Can you work these out from the drawing? Everything is in mm from the part's minimum corner. A direction names the side the tool comes from. Give positions to 0.01 mm unless a question says otherwise; leave off trailing zeros. Loops run counter-clockwise (first coordinate to the right, second up) from the corner with the lowest first, then second, coordinate; pieces in that order, holes last. Notation, with made-up numbers: (48, 48) -> (82, 48) arc R6 cw to (82, 52) -> close; hole circle Ø10 at (33.5, 2.5). An arc over 180 degrees is marked (long way). Write item = value, one per line. Start each with the question number.
1) I want a section at A-A (y = 2). List the corners of the cut face in (x, z) for me.
2) I want a section at B-B (x = 10). List the corners of the cut face in (y, z) for me, and give its area (3 significant figures).
3) I'm going to push flat-ended pins straight in: pin 1 Ø12 at (x, z) = (41.5, 8) entering from -Y; pin 2 Ø0.9 at (y, z) = (1.5, 19) entering from +X. Where does each tip first touch, or does it pass through?
4) On a 3-axis mill with a long thin cutter (end or side, diameter ignored), from which of +Z, -Z, +X, -X, +Y, -Y can I reach the whole of each face in a straight line? I mean the marked faces 1, 2 and 3. Say none if no direction works.
5) If we mould it in two halves opening along X, with no side actions, what happens to the marked faces 4, 5, 6 and 7? For each: +X half, -X half, draft (parallel to the pull), parting line (faces both ways), or undercut.
6) I need wall thicknesses on probe 1 along X at (y, z) = (0.35, 6); probe 2 along Z at (x, y) = (8, 0.9); probe 3 along Z at (x, y) = (39.5, 2.25). Which ranges of each line are inside material? Lowest first, please. Write a range as from..to.
7) I want a section at C-C (z = 22). List the corners of the cut face in (x, y) for me, and give its area (3 significant figures).
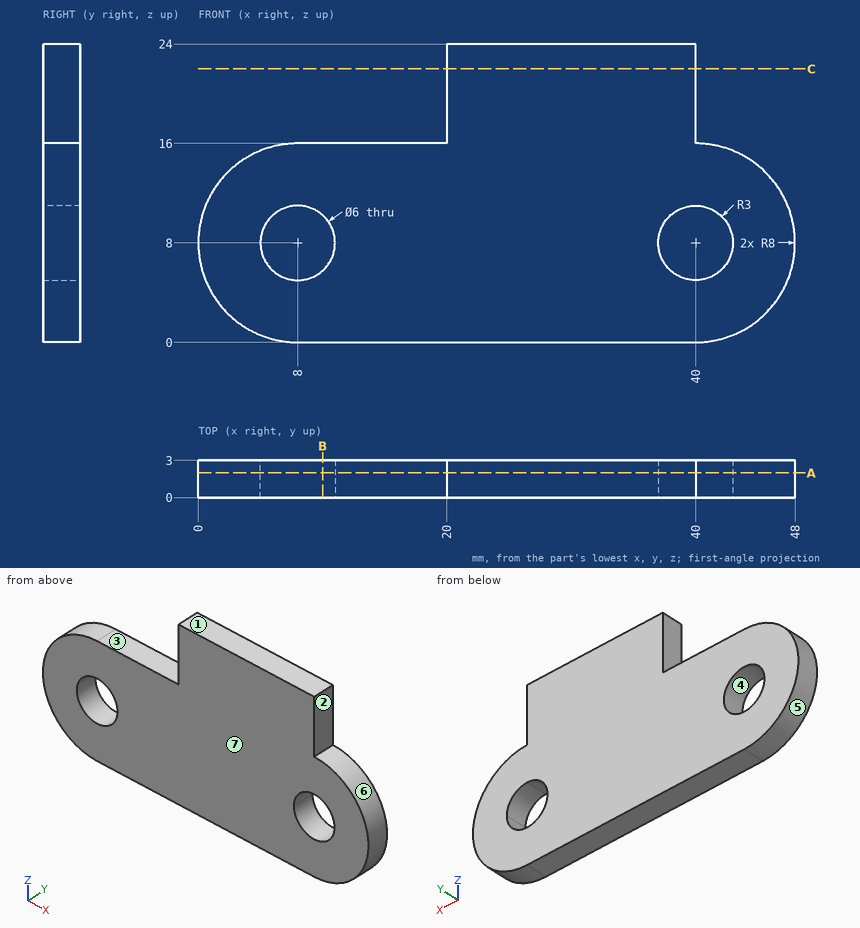
Answer list:
q1.outline = (8, 0) -> (40, 0) arc R8 ccw to (40, 16) -> (40, 24) -> (20, 24) -> (20, 16) -> (8, 16) arc R8 ccw to start; hole circle Ø6 at (8, 8); hole circle Ø6 at (40, 8)
q2.outline = (0, 0) -> (3, 0) -> (3, 5.76) -> (0, 5.76) -> close; (0, 10.24) -> (3, 10.24) -> (3, 16) -> (0, 16) -> close
q2.area = 34.6 mm^2
q3.pin_1 = 0
q3.pin_2 = 40
q4.face_1 = +Z, +X, -X, +Y, -Y
q4.face_2 = +Z, +X, +Y, -Y
q4.face_3 = +Z, -X, +Y, -Y
q5.face_4 = undercut
q5.face_5 = -X half
q5.face_6 = +X half
q5.face_7 = draft
q6.probe_1 = 0.25..5.76, 10.24..37.76, 42.24..47.75
q6.probe_2 = 0..5, 11..16
q6.probe_3 = 0..5.04, 10.96..24
q7.outline = (20, 0) -> (40, 0) -> (40, 3) -> (20, 3) -> close
q7.area = 60.0 mm^2
